```python
from build123d import *


with BuildPart() as part:
    # Sketch1 → Revolve1 (revolve)
    with BuildSketch(Plane(origin=(0, 0, 0), x_dir=(0, 0, -1), z_dir=(1, 0, 0))):
        with BuildLine():
            Line((14.859, 4.6863), (15.494, 4.6863))
            ThreePointArc((15.494, 4.6863), (16.032815367, 4.463115367), (16.256, 3.9243))
            Line((16.256, 3.9243), (16.256, 3.556))
            Line((16.256, 3.556), (15.875, 3.175))
            Line((15.875, 3.175), (3.609979933, 3.175))
            Line((3.609979933, 3.175), (3.609979933, 0))
            Line((3.609979933, 0), (0, 0))
            Line((0, 0), (0, 4.1656))
            Line((0, 4.1656), (1.806222222, 4.1656))
            Line((1.806222222, 4.1656), (3.609979933, 5.207))
            Line((3.609979933, 5.207), (13.843, 5.207))
            Line((13.843, 5.207), (13.843, 4.21767))
            Line((13.843, 4.21767), (14.859, 4.21767))
            Line((14.859, 4.21767), (14.859, 4.6863))
        make_face()
    revolve(axis=Axis((0, 0, 0), (0, 0, -1)))


solid = part.part
```
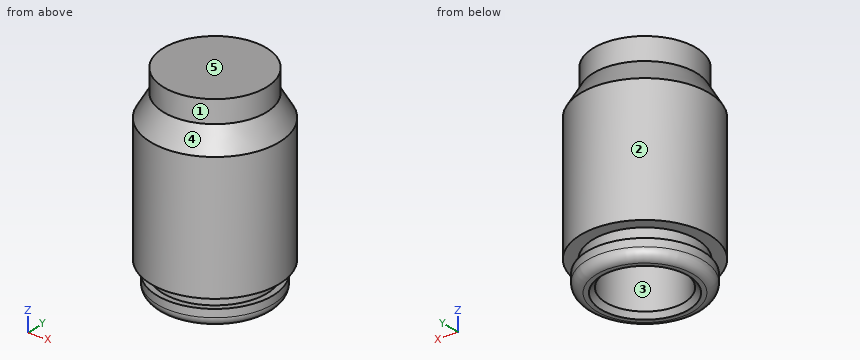
The model under review builds one solid part; all positions refer to its coordinate system, in mm. Face numbers are marked on the shaded views. A direction names the side the tool comes from. Give positions to 0.01 mm unless a question says otherwise; leave off trailing zeros. Write each loop counter-clockwise with the first axis right and the second up, starting at its lowest first coordinate (ties: lowest second). Pieces come first, ordered by that corner, then holes. Notation, with made-up numbers: M 38,25 L 54,25 A21 ccw 54,50 Z; hole C 86.25,-16 d6. An arc over 180 degrees is marked long. Write item = value, one per line. Start each with the question number.
Q1. For line 1 (X direction, y = 0, z = -9.5) (3 decimals); line 2 (Y direction, x = -2, z = -10); line 3 (Z direction, x = 1.75, y = -4), list the stretches that pass through material, from the lowest coordinate up.
Q2. Machinability: for the marked faces 1 and 2, which of the approach directions +Z, -Z, +X, -X, +Y, -Y give a long, thin tool a straight path to every point of the face, cutting with its end or side? Answer none if there is none.
Q3. Mouldability with a two-part tool opening along Y and no side actions: class the marked faces 3, 4 and 5 as released by +Y, released by -Y, zero draft, split by the parting line, or undercut.
Q4. Clearance check with flat-ended pins moving along their axes: pin 1 (3 mm diameter, centred on y = 4, z = -7, fed in from -X); pin 2 (1.5 mm diameter, centred on y = 2, z = -10.5, fed in from +X); pin 3 (3 mm diameter, centred on x = 1, y = 0.5, fed in from -Z). State where each tip first meets the part, or that it passes through.
Q5. We need section C-C (z = -11). State the section outline as (x, y) points (3 decimals).
Q6. We need section A-A (x = 0). State the section outline as (y, z) points (3 decimals).
Q7. We need section D-D (z = -1.5). State the section outline as (x, y) points.
Result set:
q1.line_1 = -5.207 to -3.175, 3.175 to 5.207
q1.line_2 = -4.81 to -2.47, 2.47 to 4.81
q1.line_3 = -16.11 to -14.86, -13.84 to -2.15
q2.face_1 = +Z
q2.face_2 = +Z, -Z
q3.face_3 = undercut
q3.face_4 = split by the parting line
q3.face_5 = zero draft
q4.pin_1 = -4.57
q4.pin_2 = 5.05
q4.pin_3 = -3.61
q5.outline = C 0,0 d10.414; hole C 0,0 d6.35
q6.outline = M -5.207,-13.843 L -4.218,-13.843 L -4.218,-14.859 L -4.686,-14.859 L -4.686,-15.494 A0.762 ccw -3.924,-16.256 L -3.556,-16.256 L -3.175,-15.875 L -3.175,-3.61 L 3.175,-3.61 L 3.175,-15.875 L 3.556,-16.256 L 3.924,-16.256 A0.762 ccw 4.686,-15.494 L 4.686,-14.859 L 4.218,-14.859 L 4.218,-13.843 L 5.207,-13.843 L 5.207,-3.61 L 4.166,-1.806 L 4.166,0 L -4.166,0 L -4.166,-1.806 L -5.207,-3.61 Z
q7.outline = C 0,0 d8.33
